Source: CAD feature listing. Evaluate the final solid. Frame: model axes, mm. Face numbers are marked on the shaded views. A direction names the side the tool comes from. Round coordinates to 2 decimals unless told otherwise and drop trailing zeros. Order: outer loops, then holes, each group sorted by start corner. A loop starts at its lowest first (then second) coordinate and runs counter-clockwise, first axis right, second up. Notation, with made-up numbers: (69, -13.5) -> (116, -13.5) arc R21 ccw to (116, 25.5) -> close; hole circle Ø3 at (-11, -15.5). An arc over 180 degrees is marked (long way). Answer as CSV lines item,"result".
from build123d import *

# Parameters (mm, degrees)
SKETCH1_W               = 50
SKETCH1_H               = 34.11
BOSS_EXTRUDE1_DEPTH     = 10
SKETCH3_W               = 41
SKETCH3_H               = 21
BOSS_EXTRUDE2_DEPTH     = 3
CUT_EXTRUDE1_DEPTH      = 32.872763059
CUT_EXTRUDE1_DEPTH_BACK = 7
SKETCH2_W               = 3.5
SKETCH2_H               = 31
SKETCH4_W               = 25
SKETCH4_H               = 21
BOSS_EXTRUDE3_DEPTH     = 20
SKETCH5_R               = 8.6
CUT_EXTRUDE2_DEPTH      = 30
SKETCH6_R               = 3.25
BOSS_EXTRUDE4_DEPTH     = 9.5
LPATTERN1_COUNT         = 3
LPATTERN1_PITCH         = 20.25
MIRROR1_COPY_1_SKETCH_R = 3.25
MIRROR1_COPY_1_DEPTH    = 9.5
MIRROR1_COPY_2_SKETCH_R = 3.25
MIRROR1_COPY_2_DEPTH    = 9.5
FILLET1_R               = 6
SKETCH7_W               = 23
SKETCH7_H               = 21
CUT_EXTRUDE3_DEPTH      = 0.5
FILLET2_R               = 6


with BuildPart() as part:
    # Sketch1 → Boss-Extrude1 (new body)
    with BuildSketch(Plane.XY):
        Rectangle(SKETCH1_W, SKETCH1_H)
    extrude(amount=BOSS_EXTRUDE1_DEPTH)

    # Sketch3 → Boss-Extrude2 (add)
    with BuildSketch(Plane(origin=(0, 0, 0), x_dir=(-1, 0, 0), z_dir=(0, 0, -1))):
        Rectangle(SKETCH3_W, SKETCH3_H)
    extrude(amount=BOSS_EXTRUDE2_DEPTH)

    # Sketch2 → Cut-Extrude1 (cut, two sides: drawn at the far end of the back side and taken through both)
    with BuildSketch(Plane(origin=(0, 0, 0), x_dir=(-1, 0, 0), z_dir=(0, 0, -1)).offset(-CUT_EXTRUDE1_DEPTH_BACK)):
        with Locations((-14.25, 0)):
            Rectangle(SKETCH2_W, SKETCH2_H)
        with Locations((14.25, 0)):
            Rectangle(SKETCH2_W, SKETCH2_H)
    extrude(amount=CUT_EXTRUDE1_DEPTH + CUT_EXTRUDE1_DEPTH_BACK, mode=Mode.SUBTRACT)

    # Sketch4 → Boss-Extrude3 (add)
    with BuildSketch(Plane(origin=(0, 0, -3), x_dir=(-1, 0, 0), z_dir=(0, 0, -1))):
        Rectangle(SKETCH4_W, SKETCH4_H)
    extrude(amount=BOSS_EXTRUDE3_DEPTH)

    # Sketch5 → Cut-Extrude2 (cut)
    with BuildSketch(Plane(origin=(0, 0, -23), x_dir=(-1, 0, 0), z_dir=(0, 0, -1))):
        Circle(SKETCH5_R)
    extrude(amount=-CUT_EXTRUDE2_DEPTH, mode=Mode.SUBTRACT)

    # Sketch6 → Boss-Extrude4 (add)
    with BuildSketch(Plane(origin=(25, 0, 0), x_dir=(0, 0, -1), z_dir=(1, 0, 0))):
        with BuildLine():
            Line((-17, 27.1), (-7, 27.1))
            Line((-7, 27.1), (-2, 17.055))
            Line((-2, 17.055), (-10, 17.055))
            Line((-10, 17.055), (-10, 14.9))
            Line((-10, 14.9), (-17, 14.9))
            ThreePointArc((-17, 14.9), (-23.1, 21), (-17, 27.1))
        make_face()
        with Locations((-17, 21)):
            Circle(SKETCH6_R, mode=Mode.SUBTRACT)
    boss_extrude4 = extrude(amount=-BOSS_EXTRUDE4_DEPTH)

    # LPattern1: Boss-Extrude4 ×3
    with Locations(*[(-i * LPATTERN1_PITCH, 0, 0) for i in range(1, LPATTERN1_COUNT)]):
        add(boss_extrude4)

    # Mirror1: Boss-Extrude4 across plane
    add(boss_extrude4.mirror(Plane.ZX))

    # Mirror1 copy 1 sketch → Mirror1 copy 1 (add)
    with BuildSketch(Plane(origin=(4.75, 0, 0), x_dir=(0, 0, -1), z_dir=(1, 0, 0))):
        with BuildLine():
            Line((-17, -27.1), (-7, -27.1))
            Line((-7, -27.1), (-2, -17.055))
            Line((-2, -17.055), (-10, -17.055))
            Line((-10, -17.055), (-10, -14.9))
            Line((-10, -14.9), (-17, -14.9))
            ThreePointArc((-17, -14.9), (-23.1, -21), (-17, -27.1))
        make_face()
        with Locations((-17, -21)):
            Circle(MIRROR1_COPY_1_SKETCH_R, mode=Mode.SUBTRACT)
    extrude(amount=-MIRROR1_COPY_1_DEPTH)

    # Mirror1 copy 2 sketch → Mirror1 copy 2 (add)
    with BuildSketch(Plane(origin=(-15.5, 0, 0), x_dir=(0, 0, -1), z_dir=(1, 0, 0))):
        with BuildLine():
            Line((-17, -27.1), (-7, -27.1))
            Line((-7, -27.1), (-2, -17.055))
            Line((-2, -17.055), (-10, -17.055))
            Line((-10, -17.055), (-10, -14.9))
            Line((-10, -14.9), (-17, -14.9))
            ThreePointArc((-17, -14.9), (-23.1, -21), (-17, -27.1))
        make_face()
        with Locations((-17, -21)):
            Circle(MIRROR1_COPY_2_SKETCH_R, mode=Mode.SUBTRACT)
    extrude(amount=-MIRROR1_COPY_2_DEPTH)

    # Fillet1
    fillet1_edges = [part.edges().sort_by_distance(p)[0] for p in [
        (20.25, 27.1, 7),
        (20.25, 14.9, 10),
        (0, 27.1, 7),
        (0, 14.9, 10),
        (-20.25, 27.1, 7),
        (-20.25, 14.9, 10),
        (20.25, -14.9, 10),
        (20.25, -27.1, 7),
        (0, -14.9, 10),
        (0, -27.1, 7),
        (-20.25, -14.9, 10),
        (-20.25, -27.1, 7),
    ]]
    fillet(fillet1_edges, radius=FILLET1_R)

    # Sketch7 → Cut-Extrude3 (cut)
    with BuildSketch(Plane(origin=(12.5, 0, 0), x_dir=(0, 0, -1), z_dir=(1, 0, 0))):
        with Locations((11.5, 0)):
            Rectangle(SKETCH7_W, SKETCH7_H)
    cut_extrude3 = extrude(amount=-CUT_EXTRUDE3_DEPTH, mode=Mode.SUBTRACT)

    # Mirror2: Cut-Extrude3 across plane
    add(cut_extrude3.mirror(Plane(origin=(0, 0, 0), x_dir=(0, 0, 1), z_dir=(1, 0, 0))), mode=Mode.SUBTRACT)

    # Fillet2
    fillet2_edges = [part.edges().sort_by_distance(p)[0] for p in [
        (10.125, 17.055, 10),
        (-10.125, 17.055, 10),
        (10.125, -17.055, 10),
        (-10.125, -17.055, 10),
    ]]
    fillet(fillet2_edges, radius=FILLET2_R)


solid = part.part
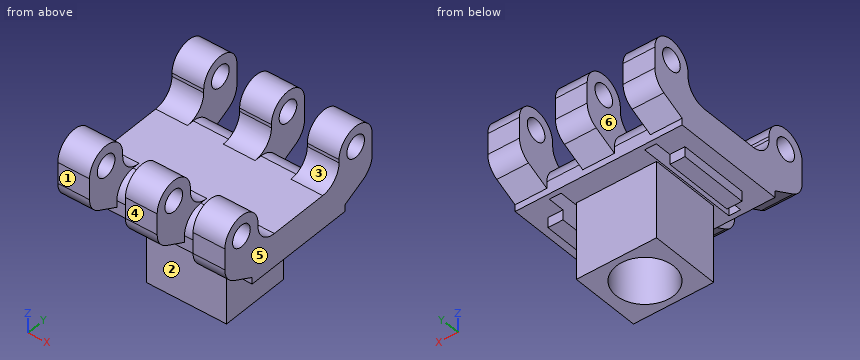
1. Section query C-C on y = 0. Return loops of the section in (x, z).
Results below:
outline,"(-25, 0) -> (-20.5, 0) -> (-20.5, -3) -> (-16, -3) -> (-16, 7) -> (-12.5, 7) -> (-12.5, 0) -> (-12, 0) -> (-12, -23) -> (-8.6, -23) -> (-8.6, 7) -> (8.6, 7) -> (8.6, -23) -> (12, -23) -> (12, 0) -> (12.5, 0) -> (12.5, 7) -> (16, 7) -> (16, -3) -> (20.5, -3) -> (20.5, 0) -> (25, 0) -> (25, 10) -> (-25, 10) -> close"
2. Pin query (flat end, axial travel): pin 1 (4 mm diameter, centred on x = 14.5, z = 2, fed in from -Y); pin 2 (6 mm diameter, centred on y = -21, z = 17, fed in from -X); pin 3 (17 mm diameter, centred on y = 4.5, z = -9, fed in from +X); pin 4 (1 mm diameter, centred on x = 4.5, y = 13, fed in from +Z). Return the tip coordinate at first contact, or that it passes through.
Results below:
pin 1,"y = -20.53"
pin 2,"through"
pin 3,"x = 20.5"
pin 4,"z = 12.15"
3. Line query: L1, parallel to X at y = -19.5, z = 7; L2, parallel to Y at x = 17, z = 17; L3, parallel to X at y = -12.5, z = 4. Output: solid intervals per line, ascending. Write a range as [from, to].
Results below:
L1,"[-25, -15.5], [-4.75, 4.75], [15.5, 25]"
L2,"[-27.1, -24.25], [-17.75, -14.9], [14.9, 17.75], [24.25, 27.1]"
L3,"[-25, -16], [-12.5, 12.5], [16, 25]"
4. Reachability of the marked faces 1, 2 and 3 from +Z, -Z, +X, -X, +Y, -Y: full face, straight path, thin tool, end or side. Return the list, or none.
Results below:
face 1,"+Z, -Z, +X, -X, -Y"
face 2,"-Z, +X, -X, -Y"
face 3,"+Z, +X, -X"
5. Section query D-D on y = 21. Return loops of the section in (x, z).
Results below:
outline,"(-25, 3.96) -> (-15.5, 3.96) -> (-15.5, 13.75) -> (-25, 13.75) -> close; (-25, 20.25) -> (-15.5, 20.25) -> (-15.5, 23.1) -> (-25, 23.1) -> close; (-4.75, 3.96) -> (4.75, 3.96) -> (4.75, 13.75) -> (-4.75, 13.75) -> close; (-4.75, 20.25) -> (4.75, 20.25) -> (4.75, 23.1) -> (-4.75, 23.1) -> close; (15.5, 3.96) -> (25, 3.96) -> (25, 13.75) -> (15.5, 13.75) -> close; (15.5, 20.25) -> (25, 20.25) -> (25, 23.1) -> (15.5, 23.1) -> close"
6. Mould query, pull axis X, two halves, no side actions, for the marked faces 4, 5 and 6. Classes: released by +X, released by -X, zero draft, split by the parting line, or undercut.
Results below:
face 4,"zero draft"
face 5,"released by +X"
face 6,"undercut"
7. Section query B-B on x = 19. Return loops of the section in (y, z) (3 decimals), and give its area (3 significant figures).
Results below:
outline,"(-27.1, 10.716) arc R6 ccw to (-23.774, 5.344) -> (-17.055, 2) -> (-17.055, 0) -> (-10.5, 0) -> (-10.5, -3) -> (10.5, -3) -> (10.5, 0) -> (17.055, 0) -> (17.055, 2) -> (23.774, 5.344) arc R6 ccw to (27.1, 10.716) -> (27.1, 17) arc R6.1 ccw to (14.9, 17) -> (14.9, 16) arc R6 cw to (8.9, 10) -> (-8.9, 10) arc R6 cw to (-14.9, 16) -> (-14.9, 17) arc R6.1 ccw to (-27.1, 17) -> close; hole circle Ø6.5 at (-21, 17); hole circle Ø6.5 at (21, 17)"
area,"747 mm2"
8. Section query A-A on z = 1. Return loops of the section in (x, y) (3 decimals), and give its area (3 significant figures).
Results below:
outline,"(-25, -17.055) -> (25, -17.055) -> (25, 17.055) -> (-25, 17.055) -> close; hole (-16, -15.5) -> (-12.5, -15.5) -> (-12.5, 15.5) -> (-16, 15.5) -> close; hole circle Ø17.2 at (0, 0); hole (12.5, -15.5) -> (16, -15.5) -> (16, 15.5) -> (12.5, 15.5) -> close"
area,"1,260 mm2"
